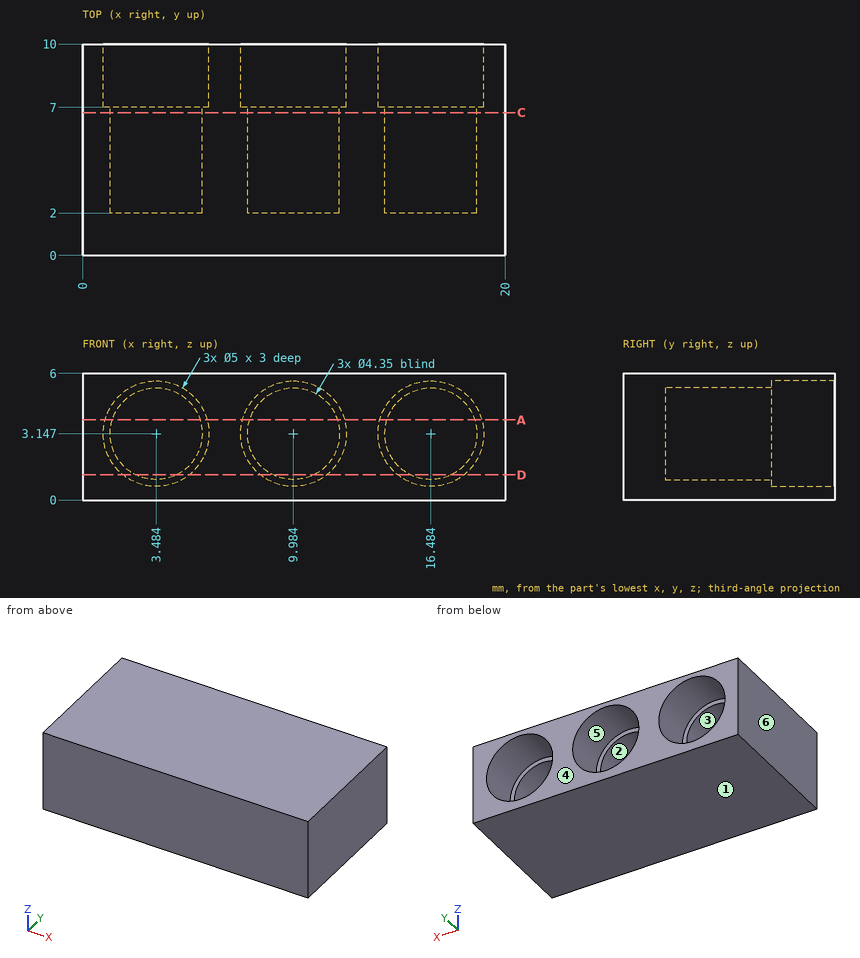
Design review of the part shown in the three views and the two pictorial views. Dimensions are in mm from the part's minimum x, y and z. A direction names the side the tool comes from. Give positions to 0.01 mm unless a question says otherwise; leave off trailing zeros. Loops run counter-clockwise (first coordinate to the right, second up) from the corner with the lowest first, then second, coordinate; pieces in that order, holes last. Notation, with made-up numbers: M -8.5,73 L 19.5,73 A10 ccw 19.5,79 Z; hole C -5.75,68 d10. An arc over 180 degrees is marked long. Write item = value, one per line.
Q1. Insertion check: pin 1 (2.5 mm diameter, centred on x = 16.5, z = 2, fed in from +Y); pin 2 (1.5 mm diameter, centred on x = 10.5, z = 2.5, fed in from +Y). Each pin has a flat end and moves straight along its axis. Give the tip position at first contact, or say it passes through.
Output values:
pin_1 = 7
pin_2 = 2
Q2. We need section A-A (z = 3.8). Give the boundary of the cut face in (x, y).
Output values:
outline = M 0,0 L 20,0 L 20,10 L 18.9,10 L 18.9,7 L 18.56,7 L 18.56,2 L 14.41,2 L 14.41,7 L 14.07,7 L 14.07,10 L 12.4,10 L 12.4,7 L 12.06,7 L 12.06,2 L 7.91,2 L 7.91,7 L 7.57,7 L 7.57,10 L 5.9,10 L 5.9,7 L 5.56,7 L 5.56,2 L 1.41,2 L 1.41,7 L 1.07,7 L 1.07,10 L 0,10 Z
Q3. We need section C-C (y = 6.75). Count the separate pieces of the cut face and the enclosed holes in it.
Output values:
separate_pieces = 1
enclosed_holes = 3
Q4. Draft analysis for pull direction Z (two halves, no side actions). For the marked faces 1, 2, 3 and 4, state which applies: +Z half, -Z half, draft (parallel to the pull), parting line (faces both ways), or undercut.
Output values:
face_1 = -Z half
face_2 = undercut
face_3 = undercut
face_4 = draft
Q5. To check wall thickness, follow line 1 (X direction, y = 8, z = 3.85) (1 decimal); line 2 (X direction, y = 3.5, z = 4.9) (1 decimal); line 3 (Z direction, x = 16.5, y = 6). State the ranges of each line that lie inside material, in increasing order. Write a range as [from, to].
Output values:
line_1 = [0, 1.1], [5.9, 7.6], [12.4, 14.1], [18.9, 20]
line_2 = [0, 2.2], [4.8, 8.7], [11.3, 15.2], [17.8, 20]
line_3 = [0, 0.97], [5.32, 6]
Q6. For the marked faces 5 and 6, list the 3-axis set-ups (+Z, -Z, +X, -X, +Y, -Y) from which the entire face can be reached by the end or side of a thin tool; tool diameter is ignored.
Output values:
face_5 = +Y
face_6 = +Z, -Z, -X, +Y, -Y
Q7. We need section D-D (z = 1.2). Give the boundary of the cut face in (x, y) (1 decimal), plus the area to 3 significant figures.
Output values:
outline = M 0,0 L 20,0 L 20,10 L 18.1,10 L 18.1,7 L 17.5,7 L 17.5,2 L 15.5,2 L 15.5,7 L 14.9,7 L 14.9,10 L 11.6,10 L 11.6,7 L 11,7 L 11,2 L 9,2 L 9,7 L 8.4,7 L 8.4,10 L 5.1,10 L 5.1,7 L 4.5,7 L 4.5,2 L 2.5,2 L 2.5,7 L 1.9,7 L 1.9,10 L 0,10 Z
area = 143 mm^2
